from build123d import *

# Parameters (mm, degrees)
F0_R     = 11.075
F1_DEPTH = 20
F3_DEPTH = 20.001
F5_DEPTH = 13.69


# Not quite as in the source:
# - a fillet or chamfer that OpenCascade refuses, or shapes differently, is made with other operations: its cross-section is extruded or revolved along the edge and cut away or added


with BuildPart() as f1:
    # F0 (on Top) → F1 (new body)
    with BuildSketch(Plane.XY):
        Circle(F0_R)
    extrude(amount=F1_DEPTH)

    # F2 (on face) → F3 (cut, through all)
    with BuildSketch(Plane.XY.offset(20)):
        with BuildLine():
            Line((4.5, 4.5), (3.5, 4.5))
            ThreePointArc((3.5, 4.5), (3.7928932188, 3.7928932188), (4.5, 3.5))
            Line((4.5, 3.5), (4.5, 4.5))
        make_face()
        with BuildLine():
            Line((-4.5, 4.5), (-3.5, 4.5))
            ThreePointArc((-3.5, 4.5), (-5.2071067812, 5.2071067812), (-4.5, 3.5))
            Line((-4.5, 3.5), (-4.5, 4.5))
        make_face()
        with BuildLine():
            ThreePointArc((-4.5, 3.5), (-3.7928932188, 3.7928932188), (-3.5, 4.5))
            Line((-3.5, 4.5), (-4.5, 4.5))
            Line((-4.5, 4.5), (-4.5, 3.5))
        make_face()
        with BuildLine():
            Line((4.5, -4.5), (4.5, -3.5))
            ThreePointArc((4.5, -3.5), (3.7928932188, -3.7928932188), (3.5, -4.5))
            Line((3.5, -4.5), (4.5, -4.5))
        make_face()
        with BuildLine():
            ThreePointArc((5.5, -4.5), (5.2071067812, -3.7928932188), (4.5, -3.5))
            Line((4.5, -3.5), (4.5, -4.5))
            Line((4.5, -4.5), (3.5, -4.5))
            ThreePointArc((3.5, -4.5), (4.5, -5.5), (5.5, -4.5))
        make_face()
        with BuildLine():
            ThreePointArc((-3.5, -4.5), (-3.7928932188, -3.7928932188), (-4.5, -3.5))
            Line((-4.5, -3.5), (-4.5, -4.5))
            Line((-4.5, -4.5), (-3.5, -4.5))
        make_face()
        with BuildLine():
            Line((-4.5, -4.5), (-4.5, -3.5))
            ThreePointArc((-4.5, -3.5), (-5.2071067812, -5.2071067812), (-3.5, -4.5))
            Line((-3.5, -4.5), (-4.5, -4.5))
        make_face()
        with BuildLine():
            ThreePointArc((5.5, 4.5), (4.5, 5.5), (3.5, 4.5))
            Line((3.5, 4.5), (4.5, 4.5))
            Line((4.5, 4.5), (4.5, 3.5))
            ThreePointArc((4.5, 3.5), (5.2071067812, 3.7928932188), (5.5, 4.5))
        make_face()
    extrude(amount=-F3_DEPTH, mode=Mode.SUBTRACT)

    # F4 (on face) → F5 (cut)
    with BuildSketch(Plane.XY.offset(20)):
        with BuildLine():
            ThreePointArc((-4.5, -3.5), (-3.7928932188, -3.7928932188), (-3.5, -4.5))
            Line((-3.5, -4.5), (-2.4, -4.5))
            ThreePointArc((-2.4, -4.5), (-3.0150757595, -3.0150757595), (-4.5, -2.4))
            Line((-4.5, -2.4), (-4.5, -3.5))
        make_face()
        with BuildLine():
            Line((-2.4, -4.5), (-3.5, -4.5))
            ThreePointArc((-3.5, -4.5), (-5.2071067812, -5.2071067812), (-4.5, -3.5))
            Line((-4.5, -3.5), (-4.5, -2.4))
            ThreePointArc((-4.5, -2.4), (-5.9849242405, -5.9849242405), (-2.4, -4.5))
        make_face()
        with BuildLine():
            ThreePointArc((4.5, -2.4), (3.0150757595, -3.0150757595), (2.4, -4.5))
            Line((2.4, -4.5), (3.5, -4.5))
            ThreePointArc((3.5, -4.5), (3.7928932188, -3.7928932188), (4.5, -3.5))
            Line((4.5, -3.5), (4.5, -2.4))
        make_face()
        with BuildLine():
            Line((3.5, -4.5), (2.4, -4.5))
            ThreePointArc((2.4, -4.5), (4.5, -6.6), (6.6, -4.5))
            ThreePointArc((6.6, -4.5), (5.9849242405, -3.0150757595), (4.5, -2.4))
            Line((4.5, -2.4), (4.5, -3.5))
            ThreePointArc((4.5, -3.5), (5.2071067812, -3.7928932188), (5.5, -4.5))
            ThreePointArc((5.5, -4.5), (4.5, -5.5), (3.5, -4.5))
        make_face()
        with BuildLine():
            ThreePointArc((-2.4, 4.5), (-5.9849242405, 5.9849242405), (-4.5, 2.4))
            Line((-4.5, 2.4), (-4.5, 3.5))
            ThreePointArc((-4.5, 3.5), (-5.2071067812, 5.2071067812), (-3.5, 4.5))
            Line((-3.5, 4.5), (-2.4, 4.5))
        make_face()
        with BuildLine():
            Line((-4.5, 3.5), (-4.5, 2.4))
            ThreePointArc((-4.5, 2.4), (-3.0150757595, 3.0150757595), (-2.4, 4.5))
            Line((-2.4, 4.5), (-3.5, 4.5))
            ThreePointArc((-3.5, 4.5), (-3.7928932188, 3.7928932188), (-4.5, 3.5))
        make_face()
        with BuildLine():
            ThreePointArc((2.4, 4.5), (3.0150757595, 3.0150757595), (4.5, 2.4))
            Line((4.5, 2.4), (4.5, 3.5))
            ThreePointArc((4.5, 3.5), (3.7928932188, 3.7928932188), (3.5, 4.5))
            Line((3.5, 4.5), (2.4, 4.5))
        make_face()
        with BuildLine():
            Line((4.5, 3.5), (4.5, 2.4))
            ThreePointArc((4.5, 2.4), (5.9849242405, 3.0150757595), (6.6, 4.5))
            ThreePointArc((6.6, 4.5), (4.5, 6.6), (2.4, 4.5))
            Line((2.4, 4.5), (3.5, 4.5))
            ThreePointArc((3.5, 4.5), (4.5, 5.5), (5.5, 4.5))
            ThreePointArc((5.5, 4.5), (5.2071067812, 3.7928932188), (4.5, 3.5))
        make_face()
        with BuildLine():
            Line((-4.5, -3.5), (-4.5, -4.5))
            Line((-4.5, -4.5), (-3.5, -4.5))
            ThreePointArc((-3.5, -4.5), (-3.7928932188, -3.7928932188), (-4.5, -3.5))
        make_face()
        with BuildLine():
            Line((-3.5, -4.5), (-4.5, -4.5))
            Line((-4.5, -4.5), (-4.5, -3.5))
            ThreePointArc((-4.5, -3.5), (-5.2071067812, -5.2071067812), (-3.5, -4.5))
        make_face()
        with BuildLine():
            ThreePointArc((4.5, -3.5), (3.7928932188, -3.7928932188), (3.5, -4.5))
            Line((3.5, -4.5), (4.5, -4.5))
            Line((4.5, -4.5), (4.5, -3.5))
        make_face()
        with BuildLine():
            Line((4.5, -4.5), (3.5, -4.5))
            ThreePointArc((3.5, -4.5), (4.5, -5.5), (5.5, -4.5))
            ThreePointArc((5.5, -4.5), (5.2071067812, -3.7928932188), (4.5, -3.5))
            Line((4.5, -3.5), (4.5, -4.5))
        make_face()
        with BuildLine():
            ThreePointArc((-3.5, 4.5), (-5.2071067812, 5.2071067812), (-4.5, 3.5))
            Line((-4.5, 3.5), (-4.5, 4.5))
            Line((-4.5, 4.5), (-3.5, 4.5))
        make_face()
        with BuildLine():
            Line((-4.5, 4.5), (-4.5, 3.5))
            ThreePointArc((-4.5, 3.5), (-3.7928932188, 3.7928932188), (-3.5, 4.5))
            Line((-3.5, 4.5), (-4.5, 4.5))
        make_face()
        with BuildLine():
            ThreePointArc((3.5, 4.5), (3.7928932188, 3.7928932188), (4.5, 3.5))
            Line((4.5, 3.5), (4.5, 4.5))
            Line((4.5, 4.5), (3.5, 4.5))
        make_face()
        with BuildLine():
            Line((4.5, 4.5), (4.5, 3.5))
            ThreePointArc((4.5, 3.5), (5.2071067812, 3.7928932188), (5.5, 4.5))
            ThreePointArc((5.5, 4.5), (4.5, 5.5), (3.5, 4.5))
            Line((3.5, 4.5), (4.5, 4.5))
        make_face()
    extrude(amount=-F5_DEPTH, mode=Mode.SUBTRACT)

    # F6: fillet of radius 11 on 1 edges, made by hand

    # F6_s1 → F6_t2 (revolve, cut)
    with BuildSketch(Plane.XZ):
        with BuildLine():
            ThreePointArc((11.075, 9), (7.8531745931, 16.7781745931), (0.075, 20))
            Line((0.075, 20), (11.075, 20))
            Line((11.075, 20), (11.075, 9))
        make_face()
    revolve(axis=Axis((0, 0, 20), (0, 0, 1)), mode=Mode.SUBTRACT)


solid = f1.part
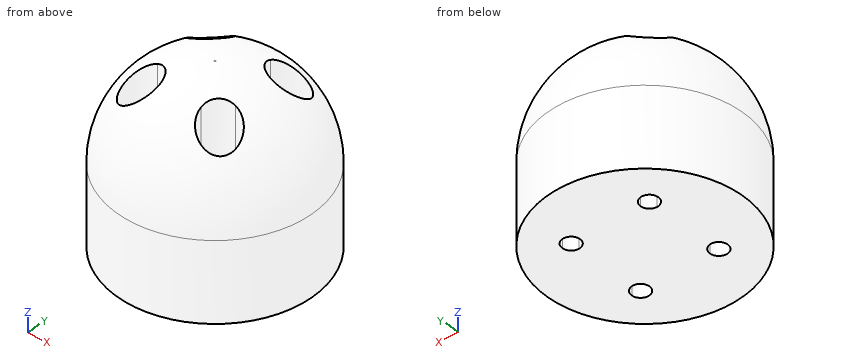
Input: part model. Units: mm. Frame: model coordinates. Give positions to 0.01 mm unless a question says otherwise; leave off trailing zeros. Write each loop counter-clockwise with the first axis right and the second up, starting at its lowest first coordinate (ties: lowest second). Pieces come first, ordered by that corner, then holes.
Q1. Section A-A, the plane z = 8. Output: boundary loops of the cut face in (x, y) (3 decimals), plus the area to 3 significant figures.
Q2. Section B-B, the plane z = 3.75. Output: boundary loops of the cut face in (x, y) (3 decimals), plus the area to 3 significant figures.
Q3. First-contact query: P1, Ø2, axis at x = 5.5, y = 2, coming from the +Z side; P2, Ø4.5, axis at x = -3.5, y = 5, coming from the +Z side; P3, Ø6, axis at x = 6, z = 6.5, coming from the -Y side. Flat tips, straight axial feed; report the tip coordinate or a pass-through.
Q4. Material intervals for probe 1 along X at (y, z) = (4.5, 9.25); probe 2 along X at (y, z) = (-4.5, 2); probe 3 along Y at (x, z) = (-4.5, 13.5), sorted ascending.
Filled in:
1. outline: circle Ø22.15 at (0, 0); hole circle Ø4.2 at (-4.5, -4.5); hole circle Ø4.2 at (-4.5, 4.5); hole circle Ø4.2 at (4.5, -4.5); hole circle Ø4.2 at (4.5, 4.5)
1. area: 330 mm2
2. outline: circle Ø22.15 at (0, 0); hole circle Ø2 at (-4.5, -4.5); hole circle Ø2 at (-4.5, 4.5); hole circle Ø2 at (4.5, -4.5); hole circle Ø2 at (4.5, 4.5)
2. area: 373 mm2
3. P1: stops at z = 18.91
3. P2: stops at z = 19.33
3. P3: stops at y = -10.66
4. probe 1: x = -10.12 to -6.6, -2.4 to 2.4, 6.6 to 10.12
4. probe 2: x = -10.12 to -5.5, -3.5 to 3.5, 5.5 to 10.12
4. probe 3: y = -9.06 to -6.6, -2.4 to 2.4, 6.6 to 9.06
